```python
from build123d import *

# Parameters (mm, degrees)
F1_DEPTH = 50.8


# Not quite as in the source:
# - the program builds the solid bodies; features that only make, move or delete a surface that nothing else refers to are left out


with BuildPart() as f1:
    # F0 (on Front) → F1 (new body, symmetric)
    with BuildSketch(Plane.XZ):
        Polygon((-63.5, -50.8), (0, -50.8), (63.5, -50.8), (63.5, 0), (101.6, 65.9911357684), (86.9353031626, 65.9911357684), (50.8, 3.4029547439), (50.8, -38.1), (0, -38.1), (-50.8, -38.1), (-50.8, 3.4029547439), (-86.9353031626, 65.9911357684), (-101.6, 65.9911357684), (-63.5, 0), align=None)
    extrude(amount=F1_DEPTH, both=True)


solid = f1.part
```
Work out the finished part from the listing and answer in its coordinate system (mm). A direction names the side the tool comes from. Coordinates: 2 decimals unless noted, no trailing zeros. Loops run counter-clockwise (first coordinate to the right, second up) from the corner with the lowest first, then second, coordinate; pieces in that order, holes last. Notation, with made-up numbers: (74, 84) - (114, 84) arc R17 ccw to (114, 113) - close; hole circle Ø7 at (-3, -32). An arc over 180 degrees is marked (long way). Use a Markdown table: item, result.
Item 1: Given pin 1 Ø15 at (y, z) = (3, -14.5) entering from +X; pin 2 Ø1.5 at (x, y) = (78, 25) entering from +Z; pin 3 Ø12.5 at (y, z) = (-21, -27) entering from -X, each flat-ended and moving along its own axis, determine where each tip first touches the part or whether it passes through.
Evaluation:
| item | result |
|---|---|
| pin 1 | stops at x = 63.5 |
| pin 2 | stops at z = 51.81 |
| pin 3 | stops at x = -63.5 |
Item 2: Find section D-D, the plane z = 29. Determine the outline of the cut face in (x, y).
Evaluation:
| item | result |
|---|---|
| outline | (-80.24, -50.8) - (-65.58, -50.8) - (-65.58, 50.8) - (-80.24, 50.8) - close; (65.58, -50.8) - (80.24, -50.8) - (80.24, 50.8) - (65.58, 50.8) - close |
Item 3: The mould has two halves that part along X. Classify faces 4 (the flat face through (-68.615, -0.711, 34.259)), 5 (the flat face through (69.1, -0.7, 35.1)), 6 (the flat face through (-63.5, -1, -25)), 7 (the flat face through (0, 50.8, -40)): +X half, -X half, draft (parallel to the pull), parting line (faces both ways), or undercut.
Evaluation:
| item | result |
|---|---|
| face 4 | undercut |
| face 5 | undercut |
| face 6 | -X half |
| face 7 | draft |
Item 4: Find section A-A, the plane z = -25.5. Determine the outline of the cut face in (x, y).
Evaluation:
| item | result |
|---|---|
| outline | (-63.5, -50.8) - (-50.8, -50.8) - (-50.8, 50.8) - (-63.5, 50.8) - close; (50.8, -50.8) - (63.5, -50.8) - (63.5, 50.8) - (50.8, 50.8) - close |
Item 5: For faces 1 (the flat face through (63.5, -1, -26)), 2 (the flat face through (-50.8, -1, -18)), 3 (the flat face through (-82.82, -0.71, 33.46)), determine the directions among +Z, -Z, +X, -X, +Y, -Y from which every point of the face is accessible in a straight line to the end or side of a thin tool.
Evaluation:
| item | result |
|---|---|
| face 1 | -Z, +X, +Y, -Y |
| face 2 | +Z, +Y, -Y |
| face 3 | -Z, -X, +Y, -Y |
Item 6: Consider probe 1 along X at (y, z) = (35, -37); probe 2 along X at (y, z) = (38, -43); probe 3 along Z at (x, y) = (10, -5). Determine where each line is inside the solid, lowest interval first. Write a range as from..to.
Evaluation:
| item | result |
|---|---|
| probe 1 | x = -63.5..-50.8, 50.8..63.5 |
| probe 2 | x = -63.5..63.5 |
| probe 3 | z = -50.8..-38.1 |
Item 7: Find section C-C, the plane x = 6. Determine the outline of the cut face in (y, z).
Evaluation:
| item | result |
|---|---|
| outline | (-50.8, -50.8) - (50.8, -50.8) - (50.8, -38.1) - (-50.8, -38.1) - close |
Item 8: Find section B-B, the plane y = 34. Determine the outline of the cut face in (x, z).
Evaluation:
| item | result |
|---|---|
| outline | (-101.6, 65.99) - (-63.5, 0) - (-63.5, -50.8) - (63.5, -50.8) - (63.5, 0) - (101.6, 65.99) - (86.94, 65.99) - (50.8, 3.4) - (50.8, -38.1) - (-50.8, -38.1) - (-50.8, 3.4) - (-86.94, 65.99) - close |
